from build123d import *

# Parameters (mm, degrees)
SKETCH_1_W          = 800
SKETCH_1_H          = 20
EXTRUDE_1_DEPTH     = 500
SKETCH_3_R          = 15
EXTRUDE_2_DEPTH     = 20
SKETCH_5_R          = 15
CUT_EXTRUDE_2_DEPTH = 1100.74273844


with BuildPart() as part:
    # 草图1 → 凸台-拉伸1 (new body)
    with BuildSketch(Plane.XY):
        Rectangle(SKETCH_1_W, SKETCH_1_H)
        with BuildLine():
            ThreePointArc((-600, 10), (-500, -22.522729151), (-400, 10))
            Line((-400, 10), (-400, -10))
            ThreePointArc((-400, -10), (-500, -42.522729151), (-600, -10))
            Line((-600, -10), (-600, 10))
        make_face()
        Polygon((-600, 10), (-781.811868577, -73.333333333), (-818.174242293, -110), (-600, -10), align=None)
    extrude(amount=EXTRUDE_1_DEPTH)

    # 草图3 → 凸台-拉伸2 (add)
    # profile 1 of 2: a face of its own
    with BuildSketch(Plane(origin=(-107.954413929, 235.52872461, 0), x_dir=(0.9090593428863094, 0.41666666666666713, 0), z_dir=(-0.41666666666666713, 0.9090593428863094, 0))):
        Polygon((-741.268939065, 0), (-541.268939065, 0), (-741.268939065, 225), align=None)
        with Locations(Location((-656.268939065, 60, 0), (0, 0, 180))):
            Circle(SKETCH_3_R, mode=Mode.SUBTRACT)
    # profile 2 of 2: a face of its own
    with BuildSketch(Plane(origin=(-107.954413929, 235.52872461, 0), x_dir=(0.9090593428863094, 0.41666666666666713, 0), z_dir=(-0.41666666666666713, 0.9090593428863094, 0))):
        Polygon((-741.268939065, -725), (-541.268939065, -500), (-741.268939065, -500), align=None)
        with Locations(Location((-656.268939065, -560, 0), (0, 0, 180))):
            Circle(SKETCH_3_R, mode=Mode.SUBTRACT)
    extrude(amount=-EXTRUDE_2_DEPTH)

    # 草图5 → 切除-拉伸2 (cut, through all)
    with BuildSketch(Plane(origin=(0, 10, 0), x_dir=(1, 0, 0), z_dir=(0, 1, 0))):
        with Locations(Location((-300, -440, 0), (0, 0, 180))):
            Circle(SKETCH_5_R)
        with Locations(Location((-300, -60, 0), (0, 0, 180))):
            Circle(SKETCH_5_R)
    extrude(amount=-CUT_EXTRUDE_2_DEPTH, mode=Mode.SUBTRACT)


solid = part.part
Design review of the part built by this model. Coordinates are the model's own, in mm. A direction names the side the tool comes from. Give positions to 0.01 mm unless a question says otherwise; leave off trailing zeros. Write each loop counter-clockwise with the first axis right and the second up, starting at its lowest first coordinate (ties: lowest second). Pieces come first, ordered by that corner, then holes. Notation, with made-up numbers: M 34.5,-22.75 L 72.5,-22.75 A23 cw 72.5,7.25 Z; hole C 3.25,68.5 d2. An arc over 180 degrees is marked long. Return JSON: item names as keys, results as strings. Group by question number.
Item 1: The part is to be moulded in two halves that separate along Z. For faces 1 (the cylindrical face through (-314.307, 0.14, 444.506)), 2 (the flat face through (-685.525, -40.047, -110.925)), 3 (the flat face through (-685, -50, 500)), 4 (the flat face through (-791, -92, 500)), say which applies: pulls with the +Z half, pulls with the -Z half, needs draft (parallel to the pull), parting line crosses it, or undercut.
Item 2: Clearance check with flat-ended pins moving along their axes: pin 1 Ø4 at (x, z) = (82, 243) entering from -Y; pin 2 Ø6 at (y, z) = (-82, 63.5) entering from -X; pin 3 Ø5 at (y, z) = (-70, 138.5) entering from +X; pin 4 Ø18 at (x, z) = (-300, 440) entering from -Y. State where each tip first meets the part, or that it passes through.
Item 3: Tool access review of faces 5 (the flat face through (-687, -51, 0)), 6 (the cylindrical face through (-501.497, -22.516, 246.5)), 7 (the flat face through (-791, -92, 0)): name each direction out of +Z, -Z, +X, -X, +Y, -Y from which nothing blocks a thin tool from reaching the whole face with its end or side.
Item 4: Take a section at D-D (z = -95.5). Give the boundary of the cut face in (x, y), plus the area to 3 significant figures.
Item 5: Take a section at C-C (x = -473). Give the boundary of the cut face in (y, z), plus the area to 4 significant figures.
Item 6: Take a section at A-A (z = 440). Give the boundary of the cut face in (x, y), plus the area to 3 significant figures.
Item 7: Take a section at B-B (x = -300). Give the boundary of the cut face in (y, z).
Item 8: Wall thickness on line 1 along Z through (x, y) = (-300, 5.5); line 2 along Y through (x, z) = (221.5, 151); line 3 along X through (y, z) = (-27.5, 296.5): over which ranges is each line inside the solid? List them lowest first.
Return value:
{
 "1": {"face 1": "undercut", "face 2": "pulls with the -Z half", "face 3": "undercut", "face 4": "pulls with the +Z half"},
 "2": {"pin 1": "stops at y = -10", "pin 2": "stops at x = -793.38", "pin 3": "stops at x = -725.45", "pin 4": "passes through"},
 "3": {"face 5": "-Y", "face 6": "+Z, -Z, +Y", "face 7": "-Z, -X, -Y"},
 "4": {"outline": "M -781.81,-73.33 L -773.48,-91.51 L -668.84,-43.55 L -677.17,-25.37 Z", "area": "2,300 mm2"},
 "5": {"outline": "M -40.36,0 L -20.36,0 L -20.36,500 L -40.36,500 Z", "area": "10,000 mm2"},
 "6": {"outline": "M -818.17,-110 L -600,-10 A170 ccw -400,-10 L -315,-10 L -315,10 L -400,10 A170 cw -600,10 L -781.81,-73.33 Z; M -285,-10 L 400,-10 L 400,10 L -285,10 Z", "area": "23,400 mm2"},
 "7": {"outline": "M -10,0 L 10,0 L 10,45 L -10,45 Z; M -10,75 L 10,75 L 10,425 L -10,425 Z; M -10,455 L 10,455 L 10,500 L -10,500 Z"},
 "8": {"line 1": "z = 0 to 45, 75 to 425, 455 to 500", "line 2": "y = -10 to 10", "line 3": "x = -681.82 to -638.18, -569.87 to -430.13"}
}
